Input: part model. Units: mm. Frame: model coordinates. Give positions to 0.01 mm unless a question says otherwise; leave off trailing zeros. Loops run counter-clockwise (first coordinate to the right, second up) from the corner with the lowest first, then second, coordinate; pieces in that order, holes last. Notation, with made-up numbers: M 56.25,25 L 106.25,25 A11 ccw 106.25,45 Z; hole C 74.25,-5 d7. An arc over 180 degrees is marked long. Return JSON: item names as keys, results as strings. Group by question number.
```python
from build123d import *

# Parameters (mm, degrees)
F0_W     = 273.05
F0_H     = 228.6
F1_DEPTH = 228.6
F3_DEPTH = 228.6
F5_DEPTH = 228.6
F7_DEPTH = 228.6


with BuildPart() as f1:
    # F0 (on Right) → F1 (new body)
    with BuildSketch(Plane.YZ):
        with Locations((136.525, 114.3)):
            Rectangle(F0_W, F0_H)
    extrude(amount=-F1_DEPTH)

    # F2 (on face) → F3 (cut, through all)
    with BuildSketch(Plane.YZ):
        Polygon((182.0333333333, 139.7), (273.05, 139.7), (273.05, 228.6), (0, 228.6), (0, 0), (91.0166666667, 0), (91.0166666667, 69.85), (182.0333333333, 69.85), align=None)
    extrude(amount=-F3_DEPTH, mode=Mode.SUBTRACT)

    # F4 (on face) → F5 (cut, through all)
    with BuildSketch(Plane.YZ):
        Polygon((201.0833333333, 50.8), (110.0666666667, 50.8), (110.0666666667, 0), (273.05, 0), (273.05, 120.65), (201.0833333333, 120.65), align=None)
    extrude(amount=-F5_DEPTH, mode=Mode.SUBTRACT)

    # F6 (on face) → F7 (cut, through all)
    with BuildSketch(Plane.YZ):
        Polygon((273.05, 139.7), (182.0333333333, 139.7), (201.0833333333, 120.65), (273.05, 120.65), align=None)
        Polygon((182.0333333333, 139.7), (182.0333333333, 69.85), (201.0833333333, 50.8), (201.0833333333, 120.65), align=None)
        Polygon((110.0666666667, 50.8), (91.0166666667, 69.85), (91.0166666667, 0), (110.0666666667, 0), align=None)
    extrude(amount=-F7_DEPTH, mode=Mode.SUBTRACT)


solid = f1.part
```
Item 1: First-contact query: pin 1 Ø4 at (x, z) = (-135, 54) entering from -Y; pin 2 Ø8 at (x, z) = (-194, 55) entering from -Y; pin 3 Ø2 at (x, y) = (-163.5, 104.5) entering from -Z. Flat tips, straight axial feed; report the tip coordinate or a pass-through.
Item 2: Section B-B, the plane z = 59.75. Return loops of the section in (x, y).
Item 3: Pull-direction query (Z, two-part tool) for faces 1 (the face through (-112.7, 100.675, 60.192)), 2 (the face through (-228.6, 145, 60)), 3 (the face through (-113, 136, 69.85)); classes: pulls with the +Z half, pulls with the -Z half, needs draft (parallel to the pull), parting line crosses it, or undercut.
Item 4: Section A-A, the plane x = -45.5. Return loops of the section in (y, z), then the cut area to 3 significant figures.
Item 5: Material intervals for line 1 (Y direction, x = -172.5, z = 56.25); line 2 (Y direction, x = -25, z = 52.5); line 3 (Z direction, x = -158, y = 109), sorted ascending. Write a range as from..to.
Answer below:
{
 "1": {"pin 1": "y = 104.87", "pin 2": "y = 101.87", "pin 3": "z = 55.37"},
 "2": {"outline": "M -228.6,101.12 L 0,101.12 L 0,192.13 L -228.6,192.13 Z"},
 "3": {"face 1": "pulls with the -Z half", "face 2": "needs draft", "face 3": "pulls with the +Z half"},
 "4": {"outline": "M 91.02,69.85 L 110.07,50.8 L 201.08,50.8 L 182.03,69.85 Z", "area": "1,730 mm^2"},
 "5": {"line 1": "104.62..195.63", "line 2": "108.37..199.38", "line 3": "51.87..69.85"}
}
